Autodesk Fusion 360 part; units mm, degrees
sketch "Skizze1" plane through (0, 0, 0) normal (0, 0, 1) x (1, 0, 0)
  line L0 (0, 0) -> (42, 0)
  line L1 (42, 0) -> (42, 25)
  line L2 (42, 25) -> (0, 25)
  line L3 (0, 25) -> (0, 0)
  dimension "d1" = 42
  dimension "d2" = 25
extrude "Extrusion1" add sketch "Skizze1" along normal blind 3
sketch "Skizze2" plane through (0, 0, 3) normal (0, 0, 1) x (-1, 0, 0)
  line L0 (0, -25) -> (0, 0)
  line L1 (0, 0) -> (-42, 0)
  line L2 (-42, 0) -> (-42, -25)
  line L3 (-42, -25) -> (0, -25)
  line L4 (-40.5, -1.5) -> (-40.5, -23.5)
  line L5 (-40.5, -23.5) -> (-1.5, -23.5)
  line L6 (-1.5, -23.5) -> (-1.5, -1.5)
  line L7 (-1.5, -1.5) -> (-40.5, -1.5)
  line L8 (-38.4799, -3.5201) -> (-38.4799, -21.4799)
  line L9 (-38.4799, -21.4799) -> (-3.5201, -21.4799)
  line L10 (-3.5201, -21.4799) -> (-3.5201, -3.5201)
  line L11 (-3.5201, -3.5201) -> (-38.4799, -3.5201)
  dimension "d6" = -1.5
  dimension "d7" = -3.5201
extrude "Extrusion2" add sketch "Skizze2" along normal blind 5 contours L4 L5 L6 L7
fillet "Abrundung1" radius 2 8 edges at (0, 25, 1.5) (1.5, 23.5, 5.5) (40.5, 23.5, 5.5) (42, 25, 1.5) (0, 0, 1.5) (1.5, 1.5, 5.5) (40.5, 1.5, 5.5) (42, 0, 1.5)
fillet "Abrundung2" radius 1.5 8 edges at (39.9142, 2.0858, 8) (40.5, 12.5, 8) (39.9142, 22.9142, 8) (21, 23.5, 8) (2.0858, 22.9142, 8) (1.5, 12.5, 8) (2.0858, 2.0858, 8) (21, 1.5, 8)
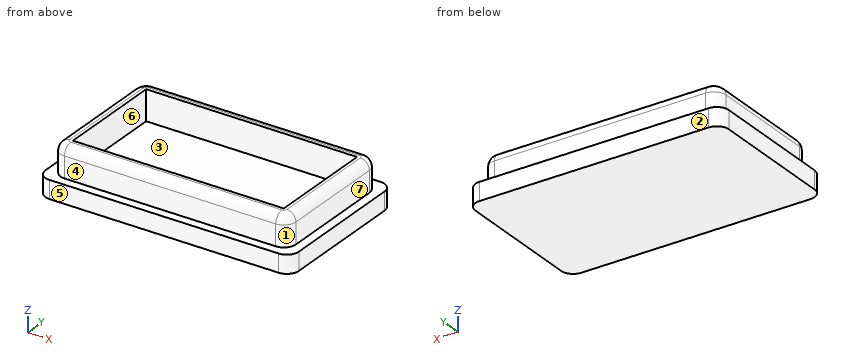
Geometry: final body of the model. Coordinates: model frame, mm. Face numbers are marked on the shaded views. A direction names the side the tool comes from. Coordinates: 2 decimals unless noted, no trailing zeros. Write each loop counter-clockwise with the first axis right and the second up, starting at its lowest first coordinate (ties: lowest second). Pieces come first, ordered by that corner, then holes. Notation, with made-up numbers: M 25.5,0.5 L 47.5,0.5 A26 cw 47.5,20.5 Z; hole C 14,17 d5. An arc over 180 degrees is marked long. Use CSV: the item, a comma, the result in double quotes. Start each with the question number.
1. First-contact query: P1, Ø3, axis at y = 8.5, z = 5, coming from the +X side; P2, Ø1, axis at x = 29.5, z = 5.5, coming from the +Y side; P3, Ø3, axis at x = 19.5, z = 5, coming from the -Y side. Flat tips, straight axial feed; report the tip coordinate or a pass-through.
2. Cut plane C-C on x = 15. Return the cut outline in (y, z), plus the area to 3 significant figures.
3. Ray query, probe 1 along X at (y, z) = (16, 6); probe 2 along Y at (x, z) = (4.5, 6); probe 3 along Z at (x, y) = (23, 11.5). Return the intervals inside material, ascending.
4. Reachability of the marked faces 1, 2, 3 and 4 from +Z, -Z, +X, -X, +Y, -Y: full face, straight path, thin tool, end or side. Return the list, or none.
5. Cut plane A-A on y = 7.25. Return the cut outline in (x, z), plus the area to 3 significant figures.
6. Mould query, pull axis X, two halves, no side actions, for the marked faces 5, 6 and 7. Classes: pulls with the +X half, pulls with the -X half, needs draft (parallel to the pull), parting line crosses it, or undercut.
7. Cut plane B-B on z = 5.75. Return the cut outline in (x, y).
Entries:
1,P1,"x = 40.5"
1,P2,"y = 23.5"
1,P3,"y = 1.5"
2,outline,"M 0,0 L 25,0 L 25,3 L 23.5,3 L 23.5,6.5 A1.5 ccw 22,8 L 21.48,8 L 21.48,3 L 3.52,3 L 3.52,8 L 3,8 A1.5 ccw 1.5,6.5 L 1.5,3 L 0,3 Z"
2,area,"94.2 mm²"
3,probe 1,"1.5 to 3.52, 38.48 to 40.5"
3,probe 2,"1.5 to 3.52, 21.48 to 23.5"
3,probe 3,"0 to 3"
4,face 1,"+Z, +X, -Y"
4,face 2,"+Z, -Z, +X, -X, +Y"
4,face 3,"+Z"
4,face 4,"+Z, +X, -X, -Y"
5,outline,"M 0,0 L 42,0 L 42,3 L 40.5,3 L 40.5,6.5 A1.5 ccw 39,8 L 38.48,8 L 38.48,3 L 3.52,3 L 3.52,8 L 3,8 A1.5 ccw 1.5,6.5 L 1.5,3 L 0,3 Z"
5,area,"145 mm²"
6,face 5,"needs draft"
6,face 6,"undercut"
6,face 7,"pulls with the +X half"
7,outline,"M 1.5,3.5 A2 ccw 3.5,1.5 L 38.5,1.5 A2 ccw 40.5,3.5 L 40.5,21.5 A2 ccw 38.5,23.5 L 3.5,23.5 A2 ccw 1.5,21.5 Z; hole M 3.52,3.52 L 38.48,3.52 L 38.48,21.48 L 3.52,21.48 Z"
